The drawing under review shows one solid part. Ordinate dimensions are in mm from its lowest x, y, z. Give positions to 0.01 mm unless a question says otherwise; leave off trailing zeros. Order: outer loops, then holes, each group sorted by start corner. A loop starts at its lowest first (then second) coordinate and runs counter-clockwise, first axis right, second up. Notation, with made-up numbers: (30.5, -18) -> (87.5, -18) arc R22 ccw to (87.5, 12) -> close; hole circle Ø2 at (0, 28.25). An arc over 180 degrees is marked (long way). One line per item, written item: value. Start each with the question number.
1) For pin 1 (15 mm diameter, centred on x = 279.4, z = 133.35, fed in from -Y), flat-tipped, find the tip position at first contact; note if it passes through.
2) Consider section A-A (x = 25.4). State the section outline as (y, z) points.
3) Wall thickness on line 1 along Z through (x, y) = (25.4, 1.75); line 2 along X through (y, z) = (2.5, 133) (1 decimal); line 3 along X through (y, z) = (6.25, 138): over which ranges is each line inside the solid? List them lowest first. Write a range as from..to.
4) Consider section B-B (z = 133.35). State the section outline as (x, y) points.
5) Consider section C-C (z = 19.05). State how many separate pieces and enclosed holes the cut face has.
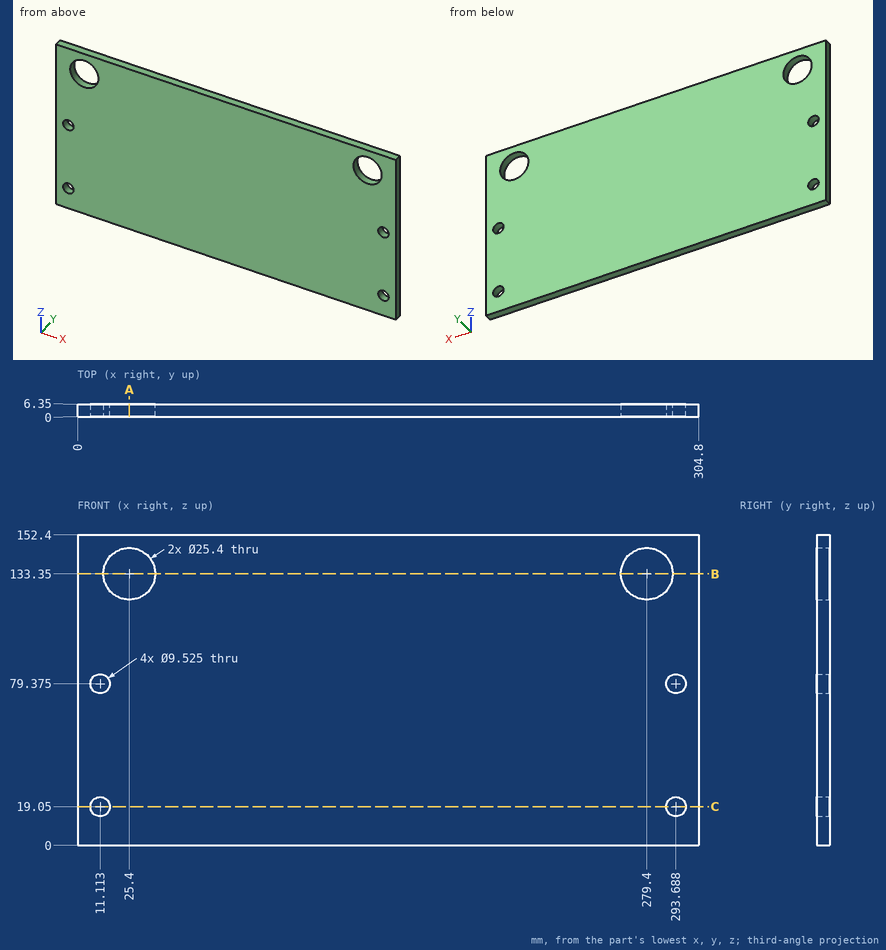
Checked values:
1. pin 1: passes through
2. outline: (0, 0) -> (6.35, 0) -> (6.35, 120.65) -> (0, 120.65) -> close; (0, 146.05) -> (6.35, 146.05) -> (6.35, 152.4) -> (0, 152.4) -> close
3. line 1: z = 0..120.65, 146.05..152.4
3. line 2: x = 0..12.7, 38.1..266.7, 292.1..304.8
3. line 3: x = 0..13.58, 37.22..267.58, 291.22..304.8
4. outline: (0, 0) -> (12.7, 0) -> (12.7, 6.35) -> (0, 6.35) -> close; (38.1, 0) -> (266.7, 0) -> (266.7, 6.35) -> (38.1, 6.35) -> close; (292.1, 0) -> (304.8, 0) -> (304.8, 6.35) -> (292.1, 6.35) -> close
5. separate pieces: 3
5. enclosed holes: 0
